```python
from build123d import *

# Parameters (mm, degrees)
F0_R          = 12.7
F1_DEPTH      = 304.8
F2_R          = 3.175
F3_DEPTH      = 40
F4_R          = 3.175
F5_DEPTH      = 40
F7_DEPTH      = 95.25
F7_DEPTH_BACK = 95.25


with BuildPart() as f1:
    # F0 (on Right) → F1 (new body)
    with BuildSketch(Plane.YZ):
        Circle(F0_R)
    extrude(amount=F1_DEPTH)

    # F2 (on face) → F3 (join)
    with BuildSketch(Plane(origin=(0, 0, 0), x_dir=(0, -1, 0), z_dir=(-1, 0, 0))):
        Circle(F2_R)
    extrude(amount=F3_DEPTH)

    # F4 (on face) → F5 (join)
    with BuildSketch(Plane.YZ.offset(304.8)):
        Circle(F4_R)
    extrude(amount=F5_DEPTH)

    # F6 (on Top) → F7 (join, two sides)
    with BuildSketch(Plane.XY) as f7_sk:
        with BuildLine():
            Line((228.6, 0), (234.95, 0))
            ThreePointArc((234.95, 0), (228.6, 6.35), (222.25, 0))
            Line((222.25, 0), (228.6, 0))
        make_face()
        with BuildLine():
            ThreePointArc((222.25, 0), (228.6, -6.35), (234.95, 0))
            Line((234.95, 0), (228.6, 0))
            Line((228.6, 0), (222.25, 0))
        make_face()
        with BuildLine():
            ThreePointArc((285.75, 0), (279.4, 6.35), (273.05, 0))
            ThreePointArc((273.05, 0), (279.4, -6.35), (285.75, 0))
        make_face()
    extrude(amount=F7_DEPTH)
    extrude(f7_sk.sketch, amount=-F7_DEPTH_BACK)


solid = f1.part
```
Build history of the part. All positions in model axes, mm. A direction names the side the tool comes from. Round coordinates to 2 decimals unless told otherwise and drop trailing zeros. Order: outer loops, then holes, each group sorted by start corner. A loop starts at its lowest first (then second) coordinate and runs counter-clockwise, first axis right, second up. Notation, with made-up numbers: (-2.75, -24) - (28.25, -24) arc R32 cw to (28.25, 14) - close; hole circle Ø2 at (68.5, 50.25). An arc over 180 degrees is marked (long way). Use a Markdown table: item, result.
1) Pull direction X, two halves, no side cores. Call faces 1 (the face through (279, 0, -95.25)), 2 (the face through (273.534, 2.432, -52.535)), 3 (the face through (304.8, 3, -3)): pulls with the +X half, pulls with the -X half, needs draft (parallel to the pull), parting line crosses it, or undercut.
Recorded:
| item | result |
|---|---|
| face 1 | needs draft |
| face 2 | undercut |
| face 3 | pulls with the +X half |
2) Tool access for faces 4 (the face through (233.64, 3.86, -52.53)), 5 (the face through (229, 0, -95.25)), 6 (the face through (279, 0, 95.25)), 7 (the face through (0, 3, -3)), 8 (the face through (233.64, 3.86, 52.53)): list every direction of +Z, -Z, +X, -X, +Y, -Y with a clear straight run to the whole face (end or side of a thin tool).
Recorded:
| item | result |
|---|---|
| face 4 | -Z |
| face 5 | -Z, +X, -X, +Y, -Y |
| face 6 | +Z, +X, -X, +Y, -Y |
| face 7 | -X |
| face 8 | +Z |
3) Saw through at B-B on x = 279.4. Write the cut outline in (y, z).
Recorded:
| item | result |
|---|---|
| outline | (-6.35, -95.25) - (6.35, -95.25) - (6.35, -11) arc R12.7 ccw to (6.35, 11) - (6.35, 95.25) - (-6.35, 95.25) - (-6.35, 11) arc R12.7 ccw to (-6.35, -11) - close |
4) Flat gauge pins, fed straight in: pin 1 Ø12.5 at (y, z) = (2.5, 4) entering from +X; pin 2 Ø3 at (x, y) = (55.5, -7) entering from -Z; pin 3 Ø2 at (x, y) = (35, 2) entering from +Z; pin 4 Ø1.5 at (x, z) = (149.5, -7.5) entering from -Y. Where does each tip first touch, or does it go through?
Recorded:
| item | result |
|---|---|
| pin 1 | stops at x = 344.8 |
| pin 2 | stops at z = -11.45 |
| pin 3 | stops at z = 12.66 |
| pin 4 | stops at y = -10.76 |
5) Saw through at C-C on x = 76. Write the cut outline in (y, z), and give its area (3 significant figures).
Recorded:
| item | result |
|---|---|
| outline | circle Ø25.4 at (0, 0) |
| area | 507 mm² |
6) Saw through at A-A on z = -42.5. Write the cut outline in (x, y).
Recorded:
| item | result |
|---|---|
| outline | circle Ø12.7 at (228.6, 0); circle Ø12.7 at (279.4, 0) |
7) Wall check: L1, parallel to X at y = -0.5, z = -44.5; L2, parallel to X at y = -4.5, z = -54.5; L3, parallel to Z at x = 301, y = -1.25. Give the ranges that are in metal, low to high.
Recorded:
| item | result |
|---|---|
| L1 | x = 222.27 to 234.93, 273.07 to 285.73 |
| L2 | x = 224.12 to 233.08, 274.92 to 283.88 |
| L3 | z = -12.64 to 12.64 |
